Read the model definition and answer for the solid it produces. Units are mm, in the model's axes. Give positions to 0.01 mm unless a question says otherwise; leave off trailing zeros. Order: outer loops, then holes, each group sorted by start corner. A loop starts at its lowest first (then second) coordinate and runs counter-clockwise, first axis right, second up. Notation, with made-up numbers: M 6,-23.75 L 41,-23.75 A10 ccw 41,-14.75 Z; hole C 52.5,-36 d3. An arc over 180 degrees is marked long. One line per item, written item: value.
from build123d import *

# Parameters (mm, degrees)
ESQUISSE1_R        = 75
ESQUISSE1_R_2      = 15
ESQUISSE1_R_3      = 5.1
ESQUISSE1_R_4      = 4.25
BOSS_EXTRU_1_DEPTH = 7.5


with BuildPart() as part:
    # Esquisse1 → Boss.-Extru.1 (new body, symmetric)
    with BuildSketch(Plane.XY):
        Circle(ESQUISSE1_R)
        Circle(ESQUISSE1_R_2, mode=Mode.SUBTRACT)
        with Locations((0, 55)):
            Circle(ESQUISSE1_R_3, mode=Mode.SUBTRACT)
        with Locations((-55, 0)):
            Circle(ESQUISSE1_R_3, mode=Mode.SUBTRACT)
        with Locations((0, -55)):
            Circle(ESQUISSE1_R_3, mode=Mode.SUBTRACT)
        with Locations((55, 0)):
            Circle(ESQUISSE1_R_3, mode=Mode.SUBTRACT)
        with Locations((10.948045608, 40.858662452)):
            Circle(ESQUISSE1_R_4, mode=Mode.SUBTRACT)
        with Locations(Location((-10.948045608, 40.858662452, 0), (0, 0, 180))):  # turned: the seam where the file's is
            Circle(ESQUISSE1_R_4, mode=Mode.SUBTRACT)
        with Locations((29.910616844, -29.910616844)):
            Circle(ESQUISSE1_R_4, mode=Mode.SUBTRACT)
        with Locations(Location((40.858662452, -10.948045608, 0), (0, 0, 180))):  # turned: the seam where the file's is
            Circle(ESQUISSE1_R_4, mode=Mode.SUBTRACT)
        with Locations((-40.858662452, -10.948045608)):
            Circle(ESQUISSE1_R_4, mode=Mode.SUBTRACT)
        with Locations(Location((-29.910616844, -29.910616844, 0), (0, 0, 180))):  # turned: the seam where the file's is
            Circle(ESQUISSE1_R_4, mode=Mode.SUBTRACT)
    extrude(amount=BOSS_EXTRU_1_DEPTH, both=True)


solid = part.part
1) Find section C-C, the plane x = 28. Write down the section's boundary in (y, z).
Reported:
outline: M -69.58,-7.5 L -33.71,-7.5 L -33.71,7.5 L -69.58,7.5 Z; M -26.11,-7.5 L 69.58,-7.5 L 69.58,7.5 L -26.11,7.5 Z
2) Find section D-D, the plane y = 55. Write down the section's boundary in (x, z).
Reported:
outline: M -50.99,-7.5 L -5.1,-7.5 L -5.1,7.5 L -50.99,7.5 Z; M 5.1,-7.5 L 50.99,-7.5 L 50.99,7.5 L 5.1,7.5 Z
3) Find section A-A, the plane x = 0. Write down the section's boundary in (y, z).
Reported:
outline: M -75,-7.5 L -60.1,-7.5 L -60.1,7.5 L -75,7.5 Z; M -49.9,-7.5 L -15,-7.5 L -15,7.5 L -49.9,7.5 Z; M 15,-7.5 L 49.9,-7.5 L 49.9,7.5 L 15,7.5 Z; M 60.1,-7.5 L 75,-7.5 L 75,7.5 L 60.1,7.5 Z
4) Each of these flat-tipped pins is pushed along its axis until it touches: pin 1 Ø5 at (x, z) = (-44.5, 5.5) entering from -Y; pin 2 Ø2 at (y, z) = (47.5, 4.5) entering from +X; pin 3 Ø1 at (y, z) = (55, -4.5) entering from -X. Where does it stop, or does it pass through?
Reported:
pin 1: stops at y = -62.14
pin 2: stops at x = 58.85
pin 3: stops at x = -51.52
5) Consider probe 1 along Y at (x, z) = (0, 1.25); probe 2 along X at (y, z) = (-8.5, 4); probe 3 along Y at (x, z) = (39, 0). Determine where each line is inside the solid, lowest interval first.
Reported:
probe 1: y = -75 to -60.1, -49.9 to -15, 15 to 49.9, 60.1 to 75
probe 2: x = -74.52 to -44.33, -37.38 to -12.36, 12.36 to 37.38, 44.33 to 74.52
probe 3: y = -64.06 to -14.77, -7.13 to 64.06
6) Determine the mould class of faces 1 (the face through (-1, -16, 7.5)), 2 (the face through (-9.764, 74.362, 0.105)), 3 (the face through (7.575, 38.273, -0.105)) for opening direction X: +X half, -X half, draft (parallel to the pull), parting line (faces both ways), or undercut.
Reported:
face 1: draft
face 2: parting line
face 3: undercut
